from build123d import *

# Parameters (mm, degrees)
BOSS_EXTRUDE1_DEPTH = 24.5
SKETCH2_W           = 103
SKETCH2_H           = 41.85
BOSS_EXTRUDE2_DEPTH = 5
SKETCH3_W           = 46.5
SKETCH3_H           = 27.85
CUT_EXTRUDE1_DEPTH  = 26
SKETCH7_W           = 8
SKETCH7_H           = 3
BOSS_EXTRUDE3_DEPTH = 8
SKETCH8_R           = 2.5
CUT_EXTRUDE2_DEPTH  = 8
SKETCH9_W           = 8
SKETCH9_H           = 3
BOSS_EXTRUDE4_DEPTH = 8
SKETCH10_R          = 2.5
CUT_EXTRUDE3_DEPTH  = 8
SKETCH12_W          = 11.5
SKETCH12_H          = 5
CUT_EXTRUDE4_DEPTH  = 8
SKETCH14_W          = 8
SKETCH14_H          = 3
BOSS_EXTRUDE5_DEPTH = 8
SKETCH15_R          = 2.5
CUT_EXTRUDE5_DEPTH  = 8
SKETCH16_W          = 8
SKETCH16_H          = 29.5
BOSS_EXTRUDE6_DEPTH = 8
SKETCH17_W          = 8
SKETCH17_H          = 29.5
BOSS_EXTRUDE7_DEPTH = 8
SKETCH18_R          = 2
CUT_EXTRUDE6_DEPTH  = 10
SKETCH20_W          = 8
SKETCH20_H          = 3
BOSS_EXTRUDE8_DEPTH = 8
SKETCH21_R          = 2.5
CUT_EXTRUDE7_DEPTH  = 8
SKETCH22_W          = 5
SKETCH22_H          = 5
CUT_EXTRUDE8_DEPTH  = 8
SKETCH23_W          = 27
SKETCH23_H          = 5
CUT_EXTRUDE9_DEPTH  = 8


with BuildPart() as part:
    # Sketch1 → Boss-Extrude1 (new body)
    with BuildSketch(Plane(origin=(0, 0, 0), x_dir=(1, 0, 0), z_dir=(0, 1, 0))):
        Polygon((0, 0), (51.5, 0), (51.5, -5), (5, -5), (5, -36.85), (51.5, -36.85), (51.5, -32.85), (56.5, -32.85), (56.5, -41.85), (0, -41.85), align=None)
    extrude(amount=BOSS_EXTRUDE1_DEPTH)

    # Sketch2 → Boss-Extrude2 (add)
    with BuildSketch(Plane.XZ):
        with Locations((51.5, 20.925)):
            Rectangle(SKETCH2_W, SKETCH2_H)
    extrude(amount=BOSS_EXTRUDE2_DEPTH)

    # Sketch3 → Cut-Extrude1 (cut)
    with BuildSketch(Plane(origin=(0, 0, 0), x_dir=(1, 0, 0), z_dir=(0, 1, 0))):
        with Locations((74.75, -18.925)):
            Rectangle(SKETCH3_W, SKETCH3_H)
    extrude(amount=-CUT_EXTRUDE1_DEPTH, mode=Mode.SUBTRACT)

    # Sketch7 → Boss-Extrude3 (add)
    with BuildSketch(Plane.XY.offset(41.85)):
        with Locations((4, -3.5)):
            Rectangle(SKETCH7_W, SKETCH7_H)
    extrude(amount=BOSS_EXTRUDE3_DEPTH)

    # Sketch8 → Cut-Extrude2 (cut)
    with BuildSketch(Plane(origin=(0, -2, 0), x_dir=(1, 0, 0), z_dir=(0, 1, 0))):
        with Locations(Location((4, -45.85, 0), (0, 0, 270))):
            Circle(SKETCH8_R)
    extrude(amount=-CUT_EXTRUDE2_DEPTH, mode=Mode.SUBTRACT)

    # Sketch9 → Boss-Extrude4 (add)
    with BuildSketch(Plane(origin=(0, 0, 0), x_dir=(-1, 0, 0), z_dir=(0, 0, -1))):
        with Locations((-99, -3.5)):
            Rectangle(SKETCH9_W, SKETCH9_H)
    extrude(amount=BOSS_EXTRUDE4_DEPTH)

    # Sketch10 → Cut-Extrude3 (cut)
    with BuildSketch(Plane(origin=(0, -2, 0), x_dir=(1, 0, 0), z_dir=(0, 1, 0))):
        with Locations(Location((99, 3.996680608, 0), (0, 0, 270))):
            Circle(SKETCH10_R)
    extrude(amount=-CUT_EXTRUDE3_DEPTH, mode=Mode.SUBTRACT)

    # Sketch12 → Cut-Extrude4 (cut)
    with BuildSketch(Plane(origin=(0, 0, 0), x_dir=(1, 0, 0), z_dir=(0, 1, 0))):
        with Locations((89.25, -2.5)):
            Rectangle(SKETCH12_W, SKETCH12_H)
    extrude(amount=-CUT_EXTRUDE4_DEPTH, mode=Mode.SUBTRACT)

    # Sketch14 → Boss-Extrude5 (add)
    with BuildSketch(Plane(origin=(0, 0, 0), x_dir=(-1, 0, 0), z_dir=(0, 0, -1))):
        with Locations((-79.5, -3.5)):
            Rectangle(SKETCH14_W, SKETCH14_H)
    extrude(amount=BOSS_EXTRUDE5_DEPTH)

    # Sketch15 → Cut-Extrude5 (cut)
    with BuildSketch(Plane(origin=(0, -2, 0), x_dir=(1, 0, 0), z_dir=(0, 1, 0))):
        with Locations(Location((79.5, 4, 0), (0, 0, 270))):
            Circle(SKETCH15_R)
    extrude(amount=-CUT_EXTRUDE5_DEPTH, mode=Mode.SUBTRACT)

    # Sketch16 → Boss-Extrude6 (add)
    with BuildSketch(Plane(origin=(0, 0, 0), x_dir=(-1, 0, 0), z_dir=(0, 0, -1))):
        with Locations((-44.5, 9.75)):
            Rectangle(SKETCH16_W, SKETCH16_H)
    extrude(amount=BOSS_EXTRUDE6_DEPTH)

    # Sketch17 → Boss-Extrude7 (add)
    with BuildSketch(Plane.XY.offset(41.85)):
        with Locations((44.5, 9.75)):
            Rectangle(SKETCH17_W, SKETCH17_H)
    extrude(amount=BOSS_EXTRUDE7_DEPTH)

    # Sketch18 → Cut-Extrude6 (cut)
    with BuildSketch(Plane(origin=(0, 24.5, 0), x_dir=(1, 0, 0), z_dir=(0, 1, 0))):
        with Locations(Location((44.5, 4, 0), (0, 0, 270))):
            Circle(SKETCH18_R)
        with Locations(Location((44.5, -45.85, 0), (0, 0, 270))):
            Circle(SKETCH18_R)
    extrude(amount=-CUT_EXTRUDE6_DEPTH, mode=Mode.SUBTRACT)

    # Sketch20 → Boss-Extrude8 (add)
    with BuildSketch(Plane(origin=(0, 0, -8), x_dir=(-1, 0, 0), z_dir=(0, 0, -1))):
        with Locations((-44.5, -3.5)):
            Rectangle(SKETCH20_W, SKETCH20_H)
    extrude(amount=BOSS_EXTRUDE8_DEPTH)

    # Sketch21 → Cut-Extrude7 (cut)
    with BuildSketch(Plane(origin=(0, -2, 0), x_dir=(1, 0, 0), z_dir=(0, 1, 0))):
        with Locations(Location((44.5, 12, 0), (0, 0, 180))):
            Circle(SKETCH21_R)
    extrude(amount=-CUT_EXTRUDE7_DEPTH, mode=Mode.SUBTRACT)

    # Sketch22 → Cut-Extrude8 (cut)
    with BuildSketch(Plane(origin=(0, 0, 0), x_dir=(1, 0, 0), z_dir=(0, 1, 0))):
        Polygon((103, -41.85), (103, 8), (56.5, 8), (56.5, 0), (83.5, 0), (83.5, -5), (56.5, -5), (56.5, -41.85), align=None)
        with Locations((54, -2.5)):
            Rectangle(SKETCH22_W, SKETCH22_H)
    extrude(amount=-CUT_EXTRUDE8_DEPTH, mode=Mode.SUBTRACT)


with BuildPart() as cut_extrude8_piece_1:
    # of the separate pieces the step leaves, piece 1, a body of its own (cut_extrude8_pieces)
    add(part.part.solids().sort_by_distance((51.5, 24.5, 0))[0])


with BuildPart() as cut_extrude8_piece_2:
    # of the separate pieces the step leaves, piece 2, a body of its own (cut_extrude8_pieces)
    add(part.part.solids().sort_by_distance((83.5, 0, 0))[0])

    # Sketch23 → Cut-Extrude9 (cut)
    with BuildSketch(Plane(origin=(0, 0, 0), x_dir=(1, 0, 0), z_dir=(0, 1, 0))):
        with Locations((70, -2.5)):
            Rectangle(SKETCH23_W, SKETCH23_H)
    extrude(amount=-CUT_EXTRUDE9_DEPTH, mode=Mode.SUBTRACT)


solid = cut_extrude8_piece_1.part
CAD build for the part. Positions are in the model's coordinates, mm. A direction names the side the tool comes from. Give positions to 0.01 mm unless a question says otherwise; leave off trailing zeros. Order: outer loops, then holes, each group sorted by start corner. A loop starts at its lowest first (then second) coordinate and runs counter-clockwise, first axis right, second up. Notation, with made-up numbers: (-14, 81.5) - (3, 81.5) arc R21 ccw to (3, 86.5) - close; hole circle Ø7 at (50, -1.75). An arc over 180 degrees is marked (long way). Answer in a Markdown table with one row per item.
1. Pull direction X, two halves, no side cores. Call faces 1 (the flat face through (48.5, 10, 46)), 2 (the flat face through (45, 11, -8)), 3 (the cylindrical face through (42.548, 19.57, 45.416)): pulls with the +X half, pulls with the -X half, needs draft (parallel to the pull), parting line crosses it, or undercut.
Data:
| item | result |
|---|---|
| face 1 | pulls with the +X half |
| face 2 | needs draft |
| face 3 | undercut |
2. Saw through at B-B, the plane y = 16. Give the cut face in (x, z), plus the area to 3 significant figures.
Data:
| item | result |
|---|---|
| outline | (0, 0) - (40.5, 0) - (40.5, -8) - (48.5, -8) - (48.5, 0) - (51.5, 0) - (51.5, 5) - (5, 5) - (5, 36.85) - (51.5, 36.85) - (51.5, 32.85) - (56.5, 32.85) - (56.5, 41.85) - (48.5, 41.85) - (48.5, 49.85) - (40.5, 49.85) - (40.5, 41.85) - (0, 41.85) - close; hole circle Ø4 at (44.5, -4); hole circle Ø4 at (44.5, 45.85) |
| area | 822 mm² |
3. Flat gauge pins, fed straight in: pin 1 (1.5 mm diameter, centred on x = 30.5, y = 20, fed in from +Z); pin 2 (0.9 mm diameter, centred on x = 50.5, y = 5.5, fed in from -Z); pin 3 (9 mm diameter, centred on x = 5, z = 46.5, fed in from +Y). Where does each tip first touch, or does it go through?
Data:
| item | result |
|---|---|
| pin 1 | stops at z = 41.85 |
| pin 2 | stops at z = 0 |
| pin 3 | stops at y = -2 |
4. Saw through at A-A, the plane z = 45.85. Give the cut face in (x, y).
Data:
| item | result |
|---|---|
| outline | (0, -5) - (1.5, -5) - (1.5, -2) - (0, -2) - close; (6.5, -5) - (8, -5) - (8, -2) - (6.5, -2) - close; (40.5, -5) - (48.5, -5) - (48.5, 24.5) - (46.5, 24.5) - (46.5, 14.5) - (42.5, 14.5) - (42.5, 24.5) - (40.5, 24.5) - close |
5. Tool access for faces 4 (the flat face through (48.5, 10, -4)), 5 (the cylindrical face through (42.548, 19.57, -4.434)), 6 (the flat face through (40.5, 10, -4)): list every direction of +Z, -Z, +X, -X, +Y, -Y with a clear straight run to the whole face (end or side of a thin tool).
Data:
| item | result |
|---|---|
| face 4 | -Z, +X, +Y, -Y |
| face 5 | +Y |
| face 6 | -Z, -X, +Y, -Y |
6. Saw through at C-C, the plane x = 44.5. Give the cut face in (y, z).
Data:
| item | result |
|---|---|
| outline | (-5, -16) - (-2, -16) - (-2, -14.5) - (-5, -14.5) - close; (-5, -9.5) - (-2, -9.5) - (-2, -8) - (24.5, -8) - (24.5, -6) - (14.5, -6) - (14.5, -2) - (24.5, -2) - (24.5, 5) - (0, 5) - (0, 36.85) - (24.5, 36.85) - (24.5, 43.85) - (14.5, 43.85) - (14.5, 47.85) - (24.5, 47.85) - (24.5, 49.85) - (-5, 49.85) - close |
7. Probe probe 1 along X at (y, z) = (-2.95, 45.85); probe 2 along Z at (x, y) = (45, 8.75); probe 3 along Y at (x, z) = (35, 27.5). List the from-to ranges inside material, lowest first. Write a range as [from, to].
Data:
| item | result |
|---|---|
| probe 1 | x = [0, 1.5], [6.5, 8], [40.5, 48.5] |
| probe 2 | z = [-8, 5], [36.85, 49.85] |
| probe 3 | y = [-5, 0] |
8. Saw through at D-D, the plane z = -12. Give the cut face in (x, y).
Data:
| item | result |
|---|---|
| outline | (40.5, -5) - (42, -5) - (42, -2) - (40.5, -2) - close; (47, -5) - (48.5, -5) - (48.5, -2) - (47, -2) - close |
